Verification items for the finished model (mm, model axes). Face numbers are marked on the shaded views. A direction names the side the tool comes from. Coordinates: 2 decimals unless noted, no trailing zeros. Order: outer loops, then holes, each group sorted by start corner. A loop starts at its lowest first (then second) coordinate and runs counter-clockwise, first axis right, second up. Notation, with made-up numbers: (89, -29) -> (136, -29) arc R21 cw to (136, -16) -> close; hole circle Ø6 at (16.25, -25.5). An arc over 180 degrees is marked (long way). Use CSV: the item, a comma, the result in double quotes. Start each with the question number.
1) Release check for a two-part mould opening along X. For the marked faces 4, 5, 6 and 7 record: released by +X, released by -X, zero draft, split by the parting line, or undercut.
2) Sectioned sample at A-A on x = -617.5. Record the boundary of the cut face in (y, z) (3 decimals).
3) Go/stop test with flat-tipped pins: pin 1 (2 mm diameter, centred on y = 2.5, z = 1, fed in from -X); pin 2 (1 mm diameter, centred on x = -609, z = -1.5, fed in from -Y); pin 3 (10 mm diameter, centred on x = -588, y = -31, fed in from +Z) (3 decimals); pin 4 (1 mm diameter, centred on y = -19, z = -1.5, fed in from +X). Record where each tip stops, or that it passes through.
4) Sectioned sample at C-C on x = -577. Record the boundary of the cut face in (y, z) (3 decimals), then the cut area to 3 significant figures.
5) Scan lines: line 1 along Y through (x, z) = (-581, 0.75); line 2 along Y through (x, z) = (-609.6, 1); line 3 along X through (y, z) = (-0.5, -0.5). Record each from-to range of solid material in increasing order.
6) Tool access check on the marked faces 1, 2 and 3. Record the directions out of +Z, -Z, +X, -X, +Y, -Y that give a thin tool (end or side, any length) a straight path to the whole face; none if there is none.
7) Sectioned sample at B-B on z = 0. Record the boundary of the cut face in (x, y).
8) Sectioned sample at D-D on x = -605. Record the boundary of the cut face in (y, z) (3 decimals), then the cut area to 3 significant figures.
from build123d import *

# Parameters (mm, degrees)
SKETCH1_R           = 12.573
SKETCH1_R_2         = 9.398
BOSS_EXTRUDE1_DEPTH = 3.175


with BuildPart() as part:
    # Sketch1 → Boss-Extrude1 (new body, symmetric)
    with BuildSketch(Plane.XY):
        with BuildLine():
            ThreePointArc((-578.972943543, -1.57558157), (-586.333231698, 1.301508328), (-583.456141799, 8.661796483))
            Line((-583.456141799, 8.661796483), (-565.308062523, 16.6092843))
            Line((-565.308062523, 16.6092843), (-567.855334259, 22.425976375))
            Line((-567.855334259, 22.425976375), (-610.775024162, 3.630394351))
            ThreePointArc((-610.775024162, 3.630394351), (-605.901582727, 3.129161319), (-601.589679699, 0.803401606))
            Line((-601.589679699, 0.803401606), (-578.370817834, -8.244100669))
            Line((-578.370817834, -8.244100669), (-558.277592531, 0.555214171))
            Line((-558.277592531, 0.555214171), (-560.824864268, 6.371906247))
            Line((-560.824864268, 6.371906247), (-578.972943543, -1.57558157))
        make_face()
        with BuildLine():
            Line((-578.370817834, -8.244100669), (-601.589679699, 0.803401606))
            ThreePointArc((-601.589679699, 0.803401606), (-598.22471789, -3.531900701), (-597.027, -8.887578616))
            ThreePointArc((-597.027, -8.887578616), (-598.11680147, -14.007781788), (-601.197282434, -18.240367853))
            Line((-601.197282434, -18.240367853), (-578.370817834, -8.244100669))
        make_face()
        with BuildLine():
            ThreePointArc((-601.197282434, -18.240367853), (-605.409721654, -20.741771815), (-610.258379573, -21.443328906))
            Line((-610.258379573, -21.443328906), (-566.600880762, -38.454986158))
            Line((-566.600880762, -38.454986158), (-564.295375476, -32.538302511))
            Line((-564.295375476, -32.538302511), (-582.755428455, -25.34512602))
            ThreePointArc((-582.755428455, -25.34512602), (-585.933265412, -18.109599759), (-578.697739152, -14.931762801))
            Line((-578.697739152, -14.931762801), (-560.237686173, -22.124939293))
            Line((-560.237686173, -22.124939293), (-557.932180888, -16.208255646))
            Line((-557.932180888, -16.208255646), (-578.370817834, -8.244100669))
            Line((-578.370817834, -8.244100669), (-601.197282434, -18.240367853))
        make_face()
        with Locations((-609.6, -8.887578616)):
            Circle(SKETCH1_R)
        with Locations((-609.6, -8.887578616)):
            Circle(SKETCH1_R_2, mode=Mode.SUBTRACT)
    extrude(amount=BOSS_EXTRUDE1_DEPTH, both=True)


solid = part.part
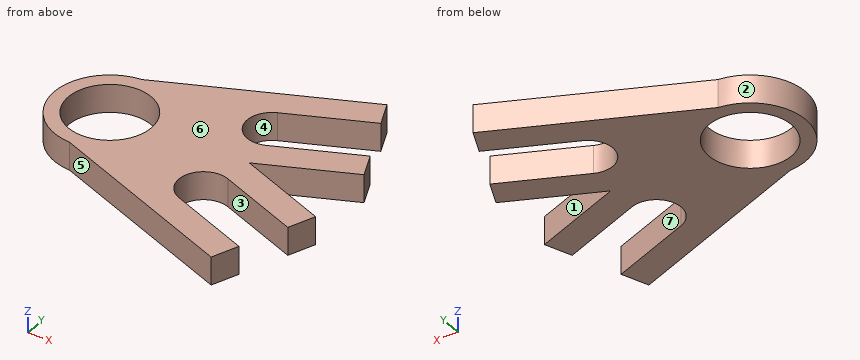
Answers follow:
1,face 4,"undercut"
1,face 5,"released by -X"
1,face 6,"zero draft"
1,face 7,"released by +X"
2,outline,"(-18.669, -3.175) -> (-13.978, -3.175) -> (-13.978, 3.175) -> (-18.669, 3.175) -> close; (-3.797, -3.175) -> (0.894, -3.175) -> (0.894, 3.175) -> (-3.797, 3.175) -> close"
3,pin 1,"stops at x = -616.68"
3,pin 2,"stops at y = -22.13"
3,pin 3,"stops at z = 3.175"
3,pin 4,"stops at x = -558.83"
4,outline,"(-34.403, -3.175) -> (-27.588, -3.175) -> (-27.588, 3.175) -> (-34.403, 3.175) -> close; (-15.593, -3.175) -> (-8.778, -3.175) -> (-8.778, 3.175) -> (-15.593, 3.175) -> close; (-7.644, -3.175) -> (-0.712, -3.175) -> (-0.712, 3.175) -> (-7.644, 3.175) -> close; (11.489, -3.175) -> (18.421, -3.175) -> (18.421, 3.175) -> (11.489, 3.175) -> close"
4,area,"175 mm²"
5,line 1,"y = -32.84 to -26.03, -14.56 to -2.04, 9.74 to 16.67"
5,line 2,"y = -21.7 to -18.29, 0.51 to 4.14"
5,line 3,"x = -618.97 to -613.84, -605.36 to -585.07, -576.52 to -560.69"
6,face 1,"+Z, -Z, +X"
6,face 2,"+Z, -Z, -X"
6,face 3,"+Z, -Z"
7,outline,"(-610.78, 3.63) arc R12.57 ccw to (-610.26, -21.44) -> (-566.6, -38.45) -> (-564.3, -32.54) -> (-582.76, -25.35) arc R5.59 cw to (-578.7, -14.93) -> (-560.24, -22.12) -> (-557.93, -16.21) -> (-578.37, -8.24) -> (-558.28, 0.56) -> (-560.82, 6.37) -> (-578.97, -1.58) arc R5.59 cw to (-583.46, 8.66) -> (-565.31, 16.61) -> (-567.86, 22.43) -> close; hole circle Ø18.8 at (-609.6, -8.89)"
8,outline,"(-23.492, -3.175) -> (-17.083, -3.175) -> (-17.083, 3.175) -> (-23.492, 3.175) -> close; (-0.692, -3.175) -> (6.159, -3.175) -> (6.159, 3.175) -> (-0.692, 3.175) -> close"
8,area,"84.2 mm²"
